Build history of the part. All positions in model axes, mm. Round coordinates to 2 decimals unless told otherwise and drop trailing zeros. Order: outer loops, then holes, each group sorted by start corner. A loop starts at its lowest first (then second) coordinate and runs counter-clockwise, first axis right, second up. Notation, with made-up numbers: (52, 62.25) -> (61, 62.25) arc R29 ccw to (61, 91.25) -> close; hole circle Ø11 at (81, -30.5). An arc over 180 degrees is marked (long way). Answer as a JSON object with one key per item and string values.
Autodesk Inventor part; units mm, degrees
ref_plane "YZ Plane" through (0, 0, 0) normal (1, 0, 0) x (0, 1, 0)
ref_plane "XZ Plane" through (0, 0, 0) normal (0, 1, 0) x (-1, 0, 0)
ref_plane "XY Plane" through (0, 0, 0) normal (0, 0, 1) x (1, 0, 0)
sketch "Sketch1" plane through (0, 0, 0) normal (0, 0, 1) x (1, 0, 0)
  line L0 (19.15, -21.15) -> (-19.15, -21.15)
  line L1 (-21.15, -19.15) -> (-21.15, 19.15)
  line L2 (-19.15, 21.15) -> (19.15, 21.15)
  line L3 (21.15, 19.15) -> (21.15, -19.15)
  line L4 (21.15, -21.15) -> (-21.15, 21.15) construction
  line L5 (-21.15, -21.15) -> (21.15, 21.15) construction
  circle A0 centre (0, 0) radius 11.25
  line L6 (15.5, -15.5) -> (-15.5, -15.5) construction
  line L7 (-15.5, -15.5) -> (-15.5, 15.5) construction
  line L8 (-15.5, 15.5) -> (15.5, 15.5) construction
  line L9 (15.5, 15.5) -> (15.5, -15.5) construction
  line L10 (15.5, -15.5) -> (-15.5, 15.5) construction
  line L11 (-15.5, -15.5) -> (15.5, 15.5) construction
  circle A1 centre (15.5, 15.5) radius 1.75
  circle A2 centre (15.5, -15.5) radius 1.75
  circle A3 centre (-15.5, -15.5) radius 1.75
  circle A4 centre (-15.5, 15.5) radius 1.75
  arc A5 (-19.15, 21.15) -> (-21.15, 19.15) centre (-19.15, 19.15) ccw
  arc A6 (21.15, 19.15) -> (19.15, 21.15) centre (19.15, 19.15) ccw
  arc A7 (19.15, -21.15) -> (21.15, -19.15) centre (19.15, -19.15) ccw
  arc A8 (-21.15, -19.15) -> (-19.15, -21.15) centre (-19.15, -19.15) ccw
  dimension "d0" = 42.3
  dimension "d1" = 42.3
  dimension "d2" = 22.5
  dimension "d3" = 31
  dimension "d4" = 31
  dimension "d5" = 3.5
  dimension "d6" = 2
extrude "Extrusion1" add sketch "Sketch1" along normal blind 2
properties part number "NEMA 17 Damper" material "Rubber, Silicone"
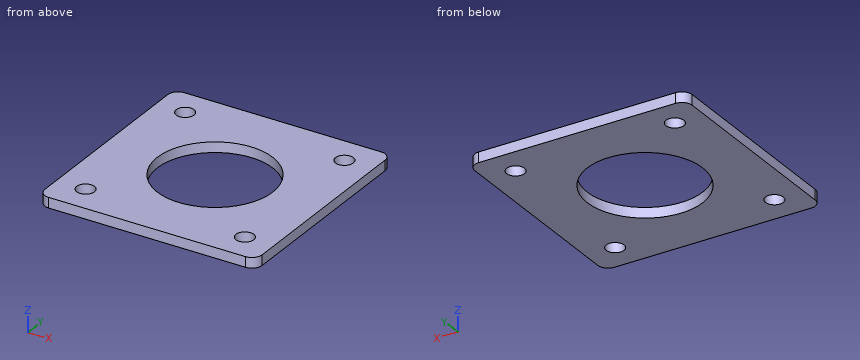
1) Cut at C-C, the plane z = 1.3. Give the cut face in (x, y).
Checked values:
{"outline": "(-21.15, -19.15) arc R2 ccw to (-19.15, -21.15) -> (19.15, -21.15) arc R2 ccw to (21.15, -19.15) -> (21.15, 19.15) arc R2 ccw to (19.15, 21.15) -> (-19.15, 21.15) arc R2 ccw to (-21.15, 19.15) -> close; hole circle Ø3.5 at (-15.5, -15.5); hole circle Ø3.5 at (-15.5, 15.5); hole circle Ø22.5 at (0, 0); hole circle Ø3.5 at (15.5, -15.5); hole circle Ø3.5 at (15.5, 15.5)"}
2) Probe L1, parallel to Y at x = 15.5, z = 0.95; L2, parallel to X at y = -15, z = 1.6; L3, parallel to Y at x = -7.5, z = 1.25. List the from-to ranges inside material, lowest first. Write a range as from..to.
Checked values:
{"L1": "y = -21.15..-17.25, -13.75..13.75, 17.25..21.15", "L2": "x = -21.15..-17.18, -13.82..13.82, 17.18..21.15", "L3": "y = -21.15..-8.39, 8.39..21.15"}
3) Cut at A-A, the plane y = 0. Give the cut face in (x, z).
Checked values:
{"outline": "(-21.15, 0) -> (-11.25, 0) -> (-11.25, 2) -> (-21.15, 2) -> close; (11.25, 0) -> (21.15, 0) -> (21.15, 2) -> (11.25, 2) -> close"}
4) Cut at D-D, the plane x = 15.5. Give the cut face in (y, z).
Checked values:
{"outline": "(-21.15, 0) -> (-17.25, 0) -> (-17.25, 2) -> (-21.15, 2) -> close; (-13.75, 0) -> (13.75, 0) -> (13.75, 2) -> (-13.75, 2) -> close; (17.25, 0) -> (21.15, 0) -> (21.15, 2) -> (17.25, 2) -> close"}
